Model file for the job. Use its own axes, mm. A direction names the side the tool comes from. Round coordinates to 2 decimals unless told otherwise and drop trailing zeros. Loops run counter-clockwise (first coordinate to the right, second up) from the corner with the lowest first, then second, coordinate; pieces in that order, holes last. Notation, with made-up numbers: (55.25, -4) -> (83.25, -4) arc R12 ccw to (83.25, 2) -> close; hole circle Ø3 at (31, 40). An arc over 180 degrees is marked (long way). Use a Markdown table: item, result.
Autodesk Inventor part; units mm, degrees
ref_plane "YZ Plane" through (0, 0, 0) normal (1, 0, 0) x (0, 1, 0)
ref_plane "XZ Plane" through (0, 0, 0) normal (0, 1, 0) x (-1, 0, 0)
ref_plane "XY Plane" through (0, 0, 0) normal (0, 0, 1) x (1, 0, 0)
sketch "Boceto1" plane through (0, 0, 0) normal (0, 1, 0) x (-1, 0, 0)
  circle A0 centre (0, 0) radius 11.25
  line L0 (-21.25, 21.25) -> (21.25, 21.25)
  line L1 (21.25, 21.25) -> (21.25, -21.25)
  line L2 (21.25, -21.25) -> (-21.25, -21.25)
  line L3 (-21.25, -21.25) -> (-21.25, 21.25)
  line L4 (-21.25, 21.25) -> (21.25, -21.25) construction
  line L5 (21.25, 21.25) -> (-21.25, -21.25) construction
  dimension "d0" = 22.5
  dimension "d1" = 42.5
  dimension "d2" = 42.5
extrude "Extrusión1" add sketch "Boceto1" along normal blind 3.5
sketch "Boceto2" plane through (0, 3.5, 0) normal (0, 1, 0) x (1, 0, 0)
  circle A0 centre (-15.5, -15.5) radius 1.7
  point P0 (0, 0)
  dimension "d5" = 15.5
  dimension "d6" = 15.5
  dimension "d7" = 3.4
extrude "Extrusión2" cut sketch "Boceto2" against normal through all
chamfer "Chaflán1" distance 1.5 angle 45 1 edges at (-17.2, 3.5, 15.5)
pattern_circular "Patrón circular1" count 4 over 360 about axis through (0, 0, 0) along (0, 1, 0) of "Extrusión2", "Chaflán1"
sketch "Boceto3" plane through (0, 3.5, 0) normal (0, 1, 0) x (1, 0, 0)
  circle A0 centre (15.5, 15.5) radius 3.2
  circle A1 centre (-15.5, -15.5) radius 3.2
  line L0 (21.25, 21.25) -> (-21.25, 21.25)
  line L1 (-21.25, 21.25) -> (-21.25, -21.25)
  line L2 (-21.25, -21.25) -> (21.25, -21.25)
  line L3 (21.25, -21.25) -> (21.25, 21.25)
  circle A2 centre (0, 0) radius 11.25
  circle A3 centre (15.5, -15.5) radius 3.2
  circle A4 centre (-15.5, 15.5) radius 3.2
  line L4 (0, -45) -> (30, -45)
  line L5 (30, -45) -> (30, 45)
  line L6 (30, 45) -> (0, 45)
  line L7 (0, 45) -> (0, -45)
  point P0 (0, -21.25)
  point P1 (0, 21.25)
  dimension "d16" = 90
  dimension "d17" = 45
  dimension "d18" = 0
  dimension "d19" = 30
extrude "Extrusión3" add sketch "Boceto3" against normal blind 17 contours L0 L7 L6 L5 L4 L2 L3
sketch "Boceto4" plane through (30, 3.5, 45) normal (1, 0, 0) x (0, 0, -1)
  circle A0 centre (10, -9.65) radius 2.1
  circle A1 centre (80, -9.65) radius 2.1
  point P0 (45, -3.5)
extrude "Extrusión4" cut sketch "Boceto4" against normal through all
properties part number "shoulder motor support"
Q1. Band-saw the part on B-B, the plane x = -15.5. Give the cut face in (y, z), plus the area to 3 significant figures.
Results list:
| item | result |
|---|---|
| outline | (0, -21.25) -> (3.5, -21.25) -> (3.5, -18.7) -> (2, -17.2) -> (0, -17.2) -> close; (0, -13.8) -> (2, -13.8) -> (3.5, -12.3) -> (3.5, 12.3) -> (2, 13.8) -> (0, 13.8) -> close; (0, 17.2) -> (2, 17.2) -> (3.5, 18.7) -> (3.5, 21.25) -> (0, 21.25) -> close |
| area | 120 mm² |
Q2. Band-saw the part on D-D, the plane y = -6.15. Give the cut face in (x, z), plus the area to 3 significant figures.
Results list:
| item | result |
|---|---|
| outline | (0, -45) -> (30, -45) -> (30, -37.1) -> (0, -37.1) -> close; (0, -32.9) -> (30, -32.9) -> (30, 32.9) -> (0, 32.9) -> (0, 21.25) -> (21.25, 21.25) -> (21.25, -21.25) -> (0, -21.25) -> close; (0, 37.1) -> (30, 37.1) -> (30, 45) -> (0, 45) -> close |
| area | 1,540 mm² |
Q3. Pull direction Z, two halves, no side cores. Call faces 1 (the face through (-16.15, 1.01, -13.93)), 2 (the face through (15, 3.5, -1)), 3 (the face through (15, -5, 45)): released by +Z, released by -Z, zero draft, split by the parting line, or undercut.
Results list:
| item | result |
|---|---|
| face 1 | undercut |
| face 2 | zero draft |
| face 3 | released by +Z |
Q4. Band-saw the part on A-A, the plane z = 15.5. Give the cut face in (x, y), plus the area to 3 significant figures.
Results list:
| item | result |
|---|---|
| outline | (-21.25, 0) -> (-17.2, 0) -> (-17.2, 2) -> (-18.7, 3.5) -> (-21.25, 3.5) -> close; (-13.8, 0) -> (13.8, 0) -> (13.8, 2) -> (12.3, 3.5) -> (-12.3, 3.5) -> (-13.8, 2) -> close; (17.2, 0) -> (21.25, 0) -> (21.25, -13.5) -> (30, -13.5) -> (30, 3.5) -> (18.7, 3.5) -> (17.2, 2) -> close |
| area | 269 mm² |
Q5. Flat gauge pins, fed straight in: pin 1 (13 mm diameter, centred on x = -7.5, z = -1.5, fed in from -Y); pin 2 (4 mm diameter, centred on y = -5, z = 25, fed in from -X); pin 3 (2.5 mm diameter, centred on x = -15.5, z = 15.5, fed in from +Y); pin 4 (1.8 mm diameter, centred on x = -9, y = 1.5, fed in from +Z). Where does each tip first touch, or does it go through?
Results list:
| item | result |
|---|---|
| pin 1 | stops at y = 0 |
| pin 2 | stops at x = 0 |
| pin 3 | passes through |
| pin 4 | stops at z = 21.25 |
Q6. Tool access for faces 4 (the face through (-9, 0, -9)), 5 (the face through (0, -5, 33)), 6 (the face through (0, -5, -33)), 7 (the face through (15.2, -6.1, -32.9)), 8 (the face through (13.93, 1.01, -16.15)): list every direction of +Z, -Z, +X, -X, +Y, -Y with a clear straight run to the whole face (end or side of a thin tool).
Results list:
| item | result |
|---|---|
| face 4 | -X, -Y |
| face 5 | +Z, -X, +Y, -Y |
| face 6 | -Z, -X, +Y, -Y |
| face 7 | +X, -X |
| face 8 | +Y, -Y |
Q7. Drill centre lines: L1, parallel to Z at x = 15.5, y = 1.35; L2, parallel to X at y = 0.55, z = 15.5; L3, parallel to Y at x = 10, z = -35. Where is each one in solid material? Low to high. Write a range as from..to.
Results list:
| item | result |
|---|---|
| L1 | z = -45..-17.2, -13.8..13.8, 17.2..45 |
| L2 | x = -21.25..-17.2, -13.8..13.8, 17.2..30 |
| L3 | y = -13.5..-8.25, -4.05..3.5 |
Q8. Band-saw the part on C-C, the plane x = 2. Give the cut face in (y, z), plus the area to 3 significant figures.
Results list:
| item | result |
|---|---|
| outline | (-13.5, -45) -> (3.5, -45) -> (3.5, -11.07) -> (0, -11.07) -> (0, -21.25) -> (-13.5, -21.25) -> close; (-13.5, 21.25) -> (0, 21.25) -> (0, 11.07) -> (3.5, 11.07) -> (3.5, 45) -> (-13.5, 45) -> close; hole circle Ø4.2 at (-6.15, -35); hole circle Ø4.2 at (-6.15, 35) |
| area | 851 mm² |
